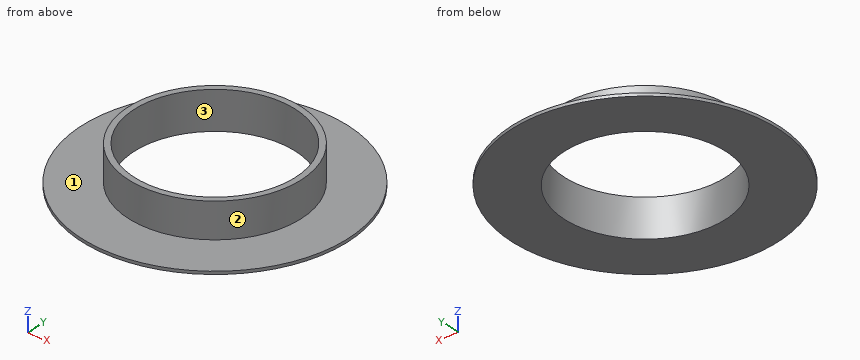
from build123d import *

# Parameters (mm, degrees)
REVOLVE_ONTO_SKETCH_ROLL_ANGLE = 90


with BuildPart() as part:
    # Sketch as drawn → Revolve (revolve)
    with BuildSketch(Plane.XY):
        Polygon((27.5, 0), (45.5, 0), (45.5, 1), (29.5, 1), (29.5, 13), (27.5, 13), align=None)
    revolve(axis=Axis((0, 0, 0), (0, 1, 0)))


with BuildPart() as part_1:
    # Revolve onto Sketch roll: moved
    add(part.part.rotate(Axis((0, 0, 0), (1, 0, 0)), REVOLVE_ONTO_SKETCH_ROLL_ANGLE))


with BuildPart() as part_2:
    # Revolve onto Sketch placement: moved
    add(part_1.part)


solid = part_2.part
The model under review builds one solid part; all positions refer to its coordinate system, in mm. Face numbers are marked on the shaded views. Round coordinates to 2 decimals unless told otherwise and drop trailing zeros. Loops run counter-clockwise (first coordinate to the right, second up) from the corner with the lowest first, then second, coordinate; pieces in that order, holes last. Notation, with made-up numbers: M -22,32.25 L 4,32.25 A16 ccw 4,57.25 Z; hole C 37,3.5 d7. An arc over 180 degrees is marked long. Answer as CSV lines item,"result". Start each with the question number.
Item 1: Insertion check: P1, Ø1, axis at x = 17, z = 7.5, coming from the +Y side; P2, Ø6, axis at x = 33, y = 1, coming from the +Z side; P3, Ø2, axis at y = 21, z = 4.5, coming from the -X side. Each pin has a flat end and moves straight along its axis. Give the tip position at first contact, or say it passes through.
Item 2: Mouldability with a two-part tool opening along Y and no side actions: class the marked faces 1, 2 and 3 as released by +Y, released by -Y, zero draft, split by the parting line, or undercut.
Item 3: Consider section D-D (x = -31). Write out the cut boundary in (y, z), then the cut area to 3 significant figures.
Item 4: Wall thickness on line 1 (Y direction, x = 0, z = 6.25); line 2 (X direction, y = 24, z = 1.5); line 3 (Z direction, x = -38, y = -23.5): over which ranges is each line inside the solid? List them lowest first. Write a range as [from, to].
Item 5: Consider section A-A (x = 0). Write out the cut boundary in (y, z).
Item 6: Consider section C-C (z = 5). Write out the cut boundary in (x, y).
Answer:
1,P1,"stops at y = 24.45"
1,P2,"stops at z = 1"
1,P3,"stops at x = -21.69"
2,face 1,"zero draft"
2,face 2,"split by the parting line"
2,face 3,"undercut"
3,outline,"M -33.31,0 L 33.31,0 L 33.31,1 L -33.31,1 Z"
3,area,"66.6 mm^2"
4,line 1,"y = [-29.5, -27.5], [27.5, 29.5]"
4,line 2,"x = [-17.15, -13.43], [13.43, 17.15]"
4,line 3,"z = [0, 1]"
5,outline,"M -45.5,0 L -27.5,0 L -27.5,13 L -29.5,13 L -29.5,1 L -45.5,1 Z; M 27.5,0 L 45.5,0 L 45.5,1 L 29.5,1 L 29.5,13 L 27.5,13 Z"
6,outline,"C 0,0 d59; hole C 0,0 d55"
